For this review, take the finished solid that the model builds, in its own axes (mm). A direction names the side the tool comes from. Round coordinates to 2 decimals unless told otherwise and drop trailing zeros. Order: outer loops, then holes, each group sorted by start corner. A loop starts at its lowest first (then second) coordinate and runs counter-clockwise, first axis right, second up. Notation, with made-up numbers: M 28.25,5 L 38.25,5 A11 cw 38.25,22 Z; hole C 63,41 d8. An arc over 180 degrees is marked long. Answer as a JSON object with one key per item and string values.
from build123d import *

# Parameters (mm, degrees)
SKETCH_1_W          = 28
SKETCH_1_H          = 24
SKETCH_1_W_2        = 3
SKETCH_1_H_2        = 10
SKETCH_1_W_3        = 10
SKETCH_1_H_3        = 3
EXTRUDE_1_DEPTH     = 3
SKETCH_2_W          = 6
SKETCH_2_H          = 3
SKETCH_2_W_2        = 3
SKETCH_2_H_2        = 2.5
SKETCH_2_W_3        = 2.5
SKETCH_2_H_3        = 6
CUT_EXTRUDE_1_DEPTH = 3
SKETCH_3_W          = 28
SKETCH_3_H          = 1
CUT_EXTRUDE_2_DEPTH = 3


with BuildPart() as part:
    # 草图1 → 凸台-拉伸1 (new body)
    with BuildSketch(Plane.XY):
        Rectangle(SKETCH_1_W, SKETCH_1_H)
        with Locations((-15.5, 0)):
            Rectangle(SKETCH_1_W_2, SKETCH_1_H_2)
        with Locations((15.5, 0)):
            Rectangle(SKETCH_1_W_2, SKETCH_1_H_2)
        with Locations((0, -13.5)):
            Rectangle(SKETCH_1_W_3, SKETCH_1_H_3)
    extrude(amount=EXTRUDE_1_DEPTH)

    # 草图2 → 切除-拉伸1 (cut)
    with BuildSketch(Plane.XY.offset(3)):
        with Locations((-14, 0)):
            Rectangle(SKETCH_2_W, SKETCH_2_H)
        with Locations((-9.5, 2.75)):
            Rectangle(SKETCH_2_W_2, SKETCH_2_H_2)
        with Locations((-9.5, 0)):
            Rectangle(SKETCH_2_W_2, SKETCH_2_H)
        with Locations((-9.5, -2.75)):
            Rectangle(SKETCH_2_W_2, SKETCH_2_H_2)
        with Locations((-6.5, 0)):
            Rectangle(SKETCH_2_W_2, SKETCH_2_H)
        with Locations((6.5, 0)):
            Rectangle(SKETCH_2_W_2, SKETCH_2_H)
        with Locations((9.5, 2.75)):
            Rectangle(SKETCH_2_W_2, SKETCH_2_H_2)
        with Locations((9.5, 0)):
            Rectangle(SKETCH_2_W_2, SKETCH_2_H)
        with Locations((9.5, -2.75)):
            Rectangle(SKETCH_2_W_2, SKETCH_2_H_2)
        with Locations((14, 0)):
            Rectangle(SKETCH_2_W, SKETCH_2_H)
        with Locations((-2.75, -7.5)):
            Rectangle(SKETCH_2_W_3, SKETCH_2_H)
        with Locations((0, -4.5)):
            Rectangle(SKETCH_2_W_2, SKETCH_2_H)
        with Locations((0, -7.5)):
            Rectangle(SKETCH_2_W_2, SKETCH_2_H)
        with Locations((2.75, -7.5)):
            Rectangle(SKETCH_2_W_3, SKETCH_2_H)
        with Locations((0, -12)):
            Rectangle(SKETCH_2_W_2, SKETCH_2_H_3)
    extrude(amount=-CUT_EXTRUDE_1_DEPTH, mode=Mode.SUBTRACT)

    # 草图3 → 切除-拉伸2 (cut)
    with BuildSketch(Plane.XY.offset(3)):
        with Locations((0, 11.5)):
            Rectangle(SKETCH_3_W, SKETCH_3_H)
    extrude(amount=-CUT_EXTRUDE_2_DEPTH, mode=Mode.SUBTRACT)


solid = part.part
1) Machinability: for faces 5 (the flat face through (6, -1.5, 2)), 6 (the flat face through (5, -14, 1)), 7 (the flat face through (-8, 3, 2)), which of the approach directions +Z, -Z, +X, -X, +Y, -Y give a long, thin tool a straight path to every point of the face, cutting with its end or side? Answer none if there is none.
Geometry check:
{"face 5": "+Z, -Z, +X", "face 6": "+Z, -Z, +X, -Y", "face 7": "+Z, -Z"}
2) Mouldability with a two-part tool opening along X and no side actions: class faces 1 (the flat face through (17, -3, 1)), 2 (the flat face through (-7, -1.5, 2)), 3 (the flat face through (11, -3, 2)), 4 (the flat face through (-1.5, -5, 2)) as +X half, -X half, draft (parallel to the pull), parting line (faces both ways), or undercut.
Geometry check:
{"face 1": "+X half", "face 2": "draft", "face 3": "undercut", "face 4": "undercut"}
3) Add section A-A on y = -8.25. State the section outline as (x, z) points, and give its area (3 significant figures).
Geometry check:
{"outline": "M -14,0 L -4,0 L -4,3 L -14,3 Z; M 4,0 L 14,0 L 14,3 L 4,3 Z", "area": "60.0 mm²"}
4) Insertion check: P1, Ø1.5, axis at y = -14, z = 1.5, coming from the +X side; P2, Ø0.9, axis at x = 16, z = 1, coming from the +Y side; P3, Ø0.9, axis at y = -11.5, z = 1, coming from the +X side. Each pin has a flat end and moves straight along its axis. Give the tip position at first contact, or say it passes through.
Geometry check:
{"P1": "stops at x = 5", "P2": "stops at y = 5", "P3": "stops at x = 14"}
5) Add section D-D on y = 8.25. State the section outline as (x, z) points.
Geometry check:
{"outline": "M -14,0 L 14,0 L 14,3 L -14,3 Z"}
6) Add section B-B on x = -3. State the section outline as (y, z) points.
Geometry check:
{"outline": "M -15,0 L -9,0 L -9,3 L -15,3 Z; M -6,0 L 11,0 L 11,3 L -6,3 Z"}
7) Add section C-C on y = 0. State the section outline as (x, z) points.
Geometry check:
{"outline": "M -5,0 L 5,0 L 5,3 L -5,3 Z"}
8) For L1, parallel to X at y = 2.5, z = 0.7; L2, parallel to X at y = -3.75, z = 1.75; L3, parallel to X at y = -13.5, z = 2.2, list the stretches that pass through material, from the lowest coordinate up.
Geometry check:
{"L1": "x = -17 to -11, -8 to 8, 11 to 17", "L2": "x = -17 to -11, -8 to -1.5, 1.5 to 8, 11 to 17", "L3": "x = -5 to -1.5, 1.5 to 5"}
